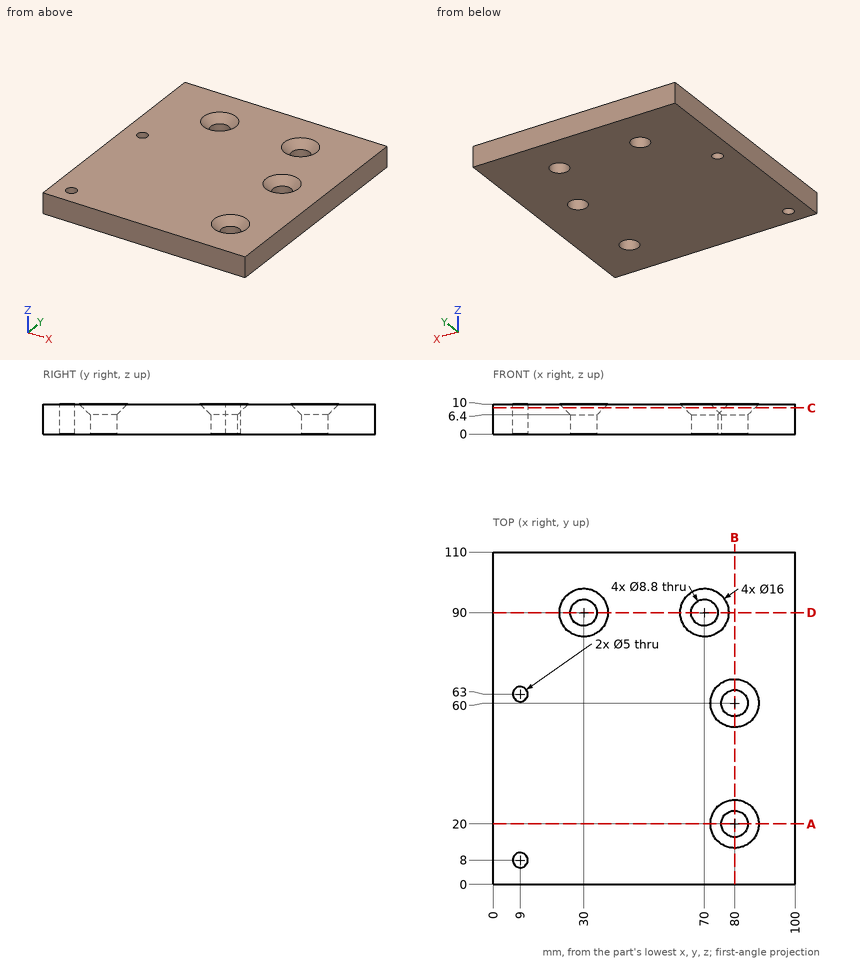
Input: dimensioned drawing with shaded views. Units: mm. Origin: part minimum x, y, z. Coordinates: 2 decimals unless noted, no trailing zeros. Order: outer loops, then holes, each group sorted by start corner. A loop starts at its lowest first (then second) coordinate and runs counter-clockwise, first axis right, second up.
(1) First-contact query: pin 1 (1 mm diameter, centred on y = 95.5, z = 4, fed in from -X); pin 2 (8 mm diameter, centred on x = 80, y = 60, fed in from -Z); pin 3 (11.5 mm diameter, centred on x = 70, y = 90, fed in from +Z). Flat tips, straight axial feed; report the tip coordinate or a pass-through.
(2) Section query A-A (y = 20). Return the cut outline in (x, z), plus the area to 3 significant figures.
(3) Section query B-B (x = 80). Return the cut outline in (y, z), plus the area to 3 significant figures.
(4) Section query D-D (y = 90). Return the cut outline in (x, z).
(5) Section query C-C (z = 8.75). Return the cut outline in (x, y).
(6) Material intervals for probe 1 along X at (y, z) = (90, 6.25); probe 2 along Y at (x, z) = (80, 4.5); probe 3 along Y at (x, z) = (7, 9.25), sorted ascending.
Solution:
1. pin 1: stops at x = 0
1. pin 2: passes through
1. pin 3: stops at z = 7.75
2. outline: (0, 0) - (75.6, 0) - (75.6, 6.4) - (72, 10) - (0, 10) - close; (84.4, 0) - (100, 0) - (100, 10) - (88, 10) - (84.4, 6.4) - close
2. area: 899 mm2
3. outline: (0, 0) - (15.6, 0) - (15.6, 6.4) - (12, 10) - (0, 10) - close; (24.4, 0) - (55.6, 0) - (55.6, 6.4) - (52, 10) - (28, 10) - (24.4, 6.4) - close; (64.4, 0) - (110, 0) - (110, 10) - (68, 10) - (64.4, 6.4) - close
3. area: 898 mm2
4. outline: (0, 0) - (25.6, 0) - (25.6, 6.4) - (22, 10) - (0, 10) - close; (34.4, 0) - (65.6, 0) - (65.6, 6.4) - (62, 10) - (38, 10) - (34.4, 6.4) - close; (74.4, 0) - (100, 0) - (100, 10) - (78, 10) - (74.4, 6.4) - close
5. outline: (0, 0) - (100, 0) - (100, 110) - (0, 110) - close; hole circle Ø5 at (9, 8); hole circle Ø5 at (9, 63); hole circle Ø13.5 at (30, 90); hole circle Ø13.5 at (70, 90); hole circle Ø13.5 at (80, 20); hole circle Ø13.5 at (80, 60)
6. probe 1: x = 0 to 25.6, 34.4 to 65.6, 74.4 to 100
6. probe 2: y = 0 to 15.6, 24.4 to 55.6, 64.4 to 110
6. probe 3: y = 0 to 6.5, 9.5 to 61.5, 64.5 to 110
